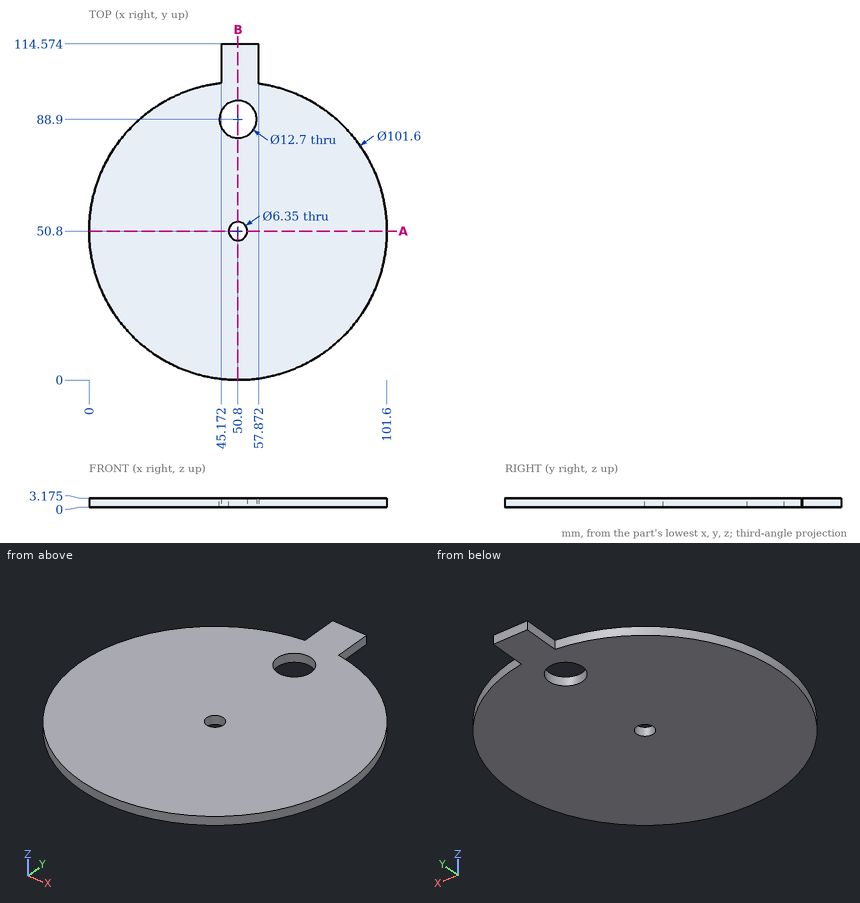
Geometry: see drawing. Coordinates: mm, zero at the bounding-box minimum. Give positions to 0.01 mm unless a question says otherwise; leave off trailing zeros. Order: outer loops, then holes, each group sorted by start corner. A loop starts at its lowest first (then second) coordinate and runs counter-clockwise, first axis right, second up. Notation, with made-up numbers: (-35.75, 40.25) -> (-4.75, 40.25) arc R27 cw to (-4.75, 71.25) -> close; hole circle Ø3 at (56, 72.25). An arc over 180 degrees is marked (long way). Write each question's results on one line, items separated by ' | '. Start each with the question number.
1) Section B-B (x = 50.8). Count the separate pieces of the cut face and the enclosed holes in it, then the cut area to 3 significant figures.
2) Line query: line 1 (X direction, y = 107, z = 0.6); line 2 (X direction, y = 90, z = 2.15) (1 decimal); line 3 (Y direction, x = 17, z = 1.95) (1 decimal). Output: solid intervals per line, ascending. Write a range as from..to.
3) First-contact query: pin 1 (1 mm diameter, centred on y = 85, z = 1, fed in from -X); pin 2 (1.6 mm diameter, centred on y = 111, z = 2, fed in from +X); pin 3 (7.5 mm diameter, centred on x = 50.8, y = 88.9, fed in from +Z); pin 4 (1 mm diameter, centred on x = 65.5, z = 1, fed in from +Y) (1 decimal). Flat tips, straight axial feed; report the tip coordinate or a pass-through.
4) Section A-A (y = 50.8). Return loops of the section in (x, z) (1 decimal).
Calculated:
1) separate pieces: 3 | enclosed holes: 0 | area: 303 mm2
2) line 1: 45.17..57.87 | line 2: 18.5..44.5, 57.1..83.1 | line 3: 12.9..88.7
3) pin 1: x = 12.79 | pin 2: x = 57.87 | pin 3: through | pin 4: y = 99.6
4) outline: (0, 0) -> (47.6, 0) -> (47.6, 3.2) -> (0, 3.2) -> close; (54, 0) -> (101.6, 0) -> (101.6, 3.2) -> (54, 3.2) -> close
